from build123d import *

# Parameters (mm, degrees)
BOSS_EXTRUDE1_DEPTH = 12.4


with BuildPart() as part:
    # Model → Boss-Extrude1 (new body)
    with BuildSketch(Plane.XY):
        Polygon((145, 35), (145, 50), (120, 50), (120, 62.4), (100, 62.4), (100, 50), (65, 50), (65, 62.4), (45, 62.4), (45, 50), (10, 50), (10, 62.4), (-10, 62.4), (-10, 50), (-45, 50), (-45, 62.4), (-65, 62.4), (-65, 50), (-100, 50), (-100, 62.4), (-120, 62.4), (-120, 50), (-145, 50), (-145, 35), (-169.8, 35), (-169.8, 15), (-145, 15), (-145, 0), (145, 0), (145, 15), (169.8, 15), (169.8, 35), align=None)
    extrude(amount=BOSS_EXTRUDE1_DEPTH)


solid = part.part
CAD build for the part. Positions are in the model's coordinates, mm. A direction names the side the tool comes from. Give positions to 0.01 mm unless a question says otherwise; leave off trailing zeros. Order: outer loops, then holes, each group sorted by start corner. A loop starts at its lowest first (then second) coordinate and runs counter-clockwise, first axis right, second up. Notation, with made-up numbers: (37.5, 80) - (52.5, 80) arc R13 cw to (52.5, 85) - close; hole circle Ø7 at (15, -15.5). An arc over 180 degrees is marked (long way). Write each question's results on one line, items separated by ' | '.
1. Pull direction X, two halves, no side cores. Call faces 5 (the face through (145, 7, 6)), 6 (the face through (-158, 15, 6)), 7 (the face through (45, 56, 6)), 8 (the face through (10, 56, 6)): released by +X, released by -X, zero draft, split by the parting line, or undercut.
Calculated:
face 5: released by +X | face 6: zero draft | face 7: undercut | face 8: undercut
2. Probe L1, parallel to X at y = 50.5, z = 5.75; L2, parallel to Y at x = -148, z = 10.25; L3, parallel to Y at x = 31.5, z = 8. List the from-to ranges inside material, lowest first. Write a range as from..to.
Calculated:
L1: x = -120..-100, -65..-45, -10..10, 45..65, 100..120 | L2: y = 15..35 | L3: y = 0..50
3. Pin check, flat tips, straight feed: pin 1 (3.5 mm diameter, centred on y = 55, z = 9, fed in from +X); pin 2 (6 mm diameter, centred on y = 11, z = 3.5, fed in from +X); pin 3 (6 mm diameter, centred on y = 56.5, z = 8, fed in from -X); pin 4 (4 mm diameter, centred on x = -36, z = 10.5, fed in from -Y). Stop position of each tip, or through.
Calculated:
pin 1: stops at x = 120 | pin 2: stops at x = 145 | pin 3: stops at x = -120 | pin 4: stops at y = 0
4. Saw through at C-C on y = 42. List the corners of the cut face in (x, z), and give its area (3 significant figures).
Calculated:
outline: (-145, 0) - (145, 0) - (145, 12.4) - (-145, 12.4) - close | area: 3,600 mm2
5. Saw through at B-B on x = -36. List the corners of the cut face in (y, z), and give its area (3 significant figures).
Calculated:
outline: (0, 0) - (50, 0) - (50, 12.4) - (0, 12.4) - close | area: 620 mm2
6. 3-axis set-ups, long thin cutter, end or side, ignore diameter. For faces 1 (the face through (-27, 50, 6)), 2 (the face through (-145, 43, 6)), 3 (the face through (157, 15, 6)), 4 (the face through (-145, 8, 6)): which of +Z, -Z, +X, -X, +Y, -Y reach the whole face in a straight line?
Calculated:
face 1: +Z, -Z, +Y | face 2: +Z, -Z, -X, +Y | face 3: +Z, -Z, +X, -Y | face 4: +Z, -Z, -X, -Y
